Input: part model. Units: mm. Frame: model coordinates. A direction names the side the tool comes from. Give positions to 0.01 mm unless a question says otherwise; leave off trailing zeros. Loops run counter-clockwise (first coordinate to the right, second up) from the corner with the lowest first, then second, coordinate; pieces in that order, holes last. Notation, with made-up numbers: (63, 72.5) -> (75, 72.5) arc R17 ccw to (75, 78.5) -> close; hole circle Ø5 at (22, 62). An arc over 180 degrees is marked (long way). Answer in a Markdown table with one row per item. Add a question column.
```python
from build123d import *

# Parameters (mm, degrees)
SKETCH_2_R      = 12.5
SKETCH_2_R_2    = 11
SKETCH_2_R_3    = 3.125
SKETCH_2_R_4    = 3.625
EXTRUDE_1_DEPTH = 1
SKETCH_2_4_R    = 3.625
SKETCH_2_4_R_2  = 3.125
EXTRUDE_2_DEPTH = 4
SKETCH_2_6_R    = 12.5
SKETCH_2_6_R_2  = 11
EXTRUDE_3_DEPTH = 11.5


with BuildPart() as part:
    # Sketch 2 → Extrude 1 (new body)
    # profile 1 of 3: a face of its own
    with BuildSketch(Plane.XY):
        Circle(SKETCH_2_R)
        Circle(SKETCH_2_R_2, mode=Mode.SUBTRACT)
    # profile 2 of 3: a face of its own
    with BuildSketch(Plane.XY):
        Circle(SKETCH_2_R_2)
        Circle(SKETCH_2_R_3, mode=Mode.SUBTRACT)
    # profile 3 of 3: a face of its own
    with BuildSketch(Plane.XY):
        Circle(SKETCH_2_R_4)
        Circle(SKETCH_2_R_3, mode=Mode.SUBTRACT)
    extrude(amount=EXTRUDE_1_DEPTH)

    # Sketch 2_4 → Extrude 2 (add)
    with BuildSketch(Plane.XY):
        Circle(SKETCH_2_4_R)
        Circle(SKETCH_2_4_R_2, mode=Mode.SUBTRACT)
    extrude(amount=EXTRUDE_2_DEPTH)

    # Sketch 2_6 → Extrude 3 (add)
    with BuildSketch(Plane.XY):
        Circle(SKETCH_2_6_R)
        Circle(SKETCH_2_6_R_2, mode=Mode.SUBTRACT)
    extrude(amount=EXTRUDE_3_DEPTH)


solid = part.part
```
1) Section D-D on z = 10.75. Output: boundary loops of the cut face in (x, y).
2) Material intervals for line 1 along Y through (x, z) = (0, 2.35) (3 decimals); line 2 along Z through (x, y) = (-3.5, -0.75); line 3 along Z through (x, y) = (6, 7), sorted ascending.
3) Reachability of faces 1 (the face through (3, -3, 0)), 2 (the face through (-3, 3, 1)) from +Z, -Z, +X, -X, +Y, -Y: full face, straight path, thin tool, end or side. Return the list, or none.
4) Pull-direction query (X, two-part tool) for faces 3 (the face through (11.923, 3.755, 5.67)), 4 (the face through (5, -10, 11.5)), 5 (the face through (1.7, -3.2, 2.5)); classes: +X half, -X half, draft (parallel to the pull), parting line (faces both ways), or undercut.
5) Section A-A on x = 0. Output: boundary loops of the cut face in (y, z) (3 decimals), and give its area (4 significant figures).
6) Pin query (flat end, axial travel): pin 1 (6 mm diameter, centred on x = 0.5, y = 0, fed in from +Z); pin 2 (1 mm diameter, centred on y = -6.5, z = 3.5, fed in from -X); pin 3 (6 mm diameter, centred on x = 4, z = 7.5, fed in from -Y). Return the tip coordinate at first contact, or that it passes through.
7) Section C-C on z = 3.5. Output: boundary loops of the cut face in (x, y) (3 decimals).
Working result:
| question | item | result |
|---|---|---|
| 1 | outline | circle Ø25 at (0, 0); hole circle Ø22 at (0, 0) |
| 2 | line 1 | y = -12.5 to -11, -3.625 to -3.125, 3.125 to 3.625, 11 to 12.5 |
| 2 | line 2 | z = 0 to 4 |
| 2 | line 3 | z = 0 to 1 |
| 3 | face 1 | -Z, +X, -X, +Y, -Y |
| 3 | face 2 | +Z |
| 4 | face 3 | parting line |
| 4 | face 4 | draft |
| 4 | face 5 | undercut |
| 5 | outline | (-12.5, 0) -> (-3.125, 0) -> (-3.125, 4) -> (-3.625, 4) -> (-3.625, 1) -> (-11, 1) -> (-11, 11.5) -> (-12.5, 11.5) -> close; (3.125, 0) -> (12.5, 0) -> (12.5, 11.5) -> (11, 11.5) -> (11, 1) -> (3.625, 1) -> (3.625, 4) -> (3.125, 4) -> close |
| 5 | area | 53.25 mm2 |
| 6 | pin 1 | stops at z = 4 |
| 6 | pin 2 | stops at x = -10.97 |
| 6 | pin 3 | stops at y = -12.46 |
| 7 | outline | circle Ø25 at (0, 0); circle Ø7.25 at (0, 0); hole circle Ø22 at (0, 0); hole circle Ø6.25 at (0, 0) |
